Can you work these out from the model? Positions are in its coordinate system, mm. Coordinates: 2 decimals unless noted, no trailing zeros. Order: outer loops, then holes, each group sorted by start corner. A loop starts at its lowest first (then second) coordinate and runs counter-clockwise, first axis right, second up. Notation, with made-up numbers: (58, 74.25) -> (66, 74.25) arc R24 ccw to (66, 101.25) -> close; hole circle Ø8 at (37, 84.25). An arc over 180 degrees is marked (long way). Answer in a Markdown table with one row per item.
Autodesk Inventor part; units mm, degrees
ref_plane "YZ Plane" through (0, 0, 0) normal (1, 0, 0) x (0, 1, 0)
ref_plane "XZ Plane" through (0, 0, 0) normal (0, 1, 0) x (-1, 0, 0)
ref_plane "XY Plane" through (0, 0, 0) normal (0, 0, 1) x (1, 0, 0)
sketch "Szkic1" plane through (0, 0, 0) normal (0, 0, 1) x (1, 0, 0)
  arc A0 (-870, 0) -> (870, 0) centre (0, 0) ccw
  line L0 (-870, 0) -> (870, 0)
  dimension "d0" = 1740
extrude "Płyta1" add sketch "Szkic1" along normal blind 3
sketch "Szkic2" plane through (0, 0, 3) normal (0, 0, 1) x (1, 0, 0)
  circle A0 centre (-780, -80) radius 25
  arc A1 (-870, 0) -> (870, 0) centre (0, 0) ccw
  dimension "d2" = 50
  dimension "d3" = 80
  dimension "d4" = 780
extrude "Wyciągnięcie proste1" cut sketch "Szkic2" against normal blind 10
chamfer "Faza1" distance 2 angle 45 1 edges at (0, 0, 0)
equation "\"d1\" = Grubość"
equation "\"PromieńGięcia\" = Grubość"
equation "\"SzerokośćGięciaPodcięcia\" = Grubość"
equation "\"GłębokośćGięciaPodcięcia\" = 0.5 * Grubość"
equation "\"RozmiarPodcięciaNarożnika\" = 4 * Grubość"
equation "\"MinimalnaPozostałość\" = 2 * Grubość"
equation "\"PromieńPrzejścia\" = PromieńGięcia"
equation "\"Rozmiar_promienia_Jacobiego\" = PromieńGięcia"
equation "\"Wielk_odstępu\" = Grubość"
properties part number "fllooor22" material "Stal nierdzewna"
(1) Suppose I cut it at C-C (x = 617). Please give me the cut outline in (y, z), and give its area (3 significant figures).
Response values:
| item | result |
|---|---|
| outline | (-613.36, 0) -> (-2, 0) -> (0, 2) -> (0, 3) -> (-613.36, 3) -> close |
| area | 1,840 mm2 |
(2) I need wall thicknesses on line 1 (Y direction, x = -780, z = 2.3); line 2 (Y direction, x = -130.5, z = 2); line 3 (X direction, y = -38.5, z = 2.2). Which ranges of each line are inside material? Lowest first, please. Write a range as [from, to].
Response values:
| item | result |
|---|---|
| line 1 | [-385.36, -105], [-55, 0] |
| line 2 | [-860.16, 0] |
| line 3 | [-869.15, 869.15] |
(3) Suppose I cut it at D-D (z = 0.8). Please give me the cut outline in (x, y), and give its area (3 significant figures).
Response values:
| item | result |
|---|---|
| outline | (-870, -1.2) arc R870 ccw to (870, -1.2) -> close; hole circle Ø50 at (-780, -80) |
| area | 1,180,000 mm2 |
(4) Will these pins go through, and if not, where does the flat tip stop? pin 1 Ø1.5 at (y, z) = (-636.5, 1.5) entering from +X; pin 2 Ø1.5 at (y, z) = (-191, 2.5) entering from +X.
Response values:
| item | result |
|---|---|
| pin 1 | x = 593.9 |
| pin 2 | x = 848.94 |
(5) Suppose I cut it at B-B (x = -780). Please give me the cut outline in (y, z), and give its area (3 significant figures).
Response values:
| item | result |
|---|---|
| outline | (-385.36, 0) -> (-105, 0) -> (-105, 3) -> (-385.36, 3) -> close; (-55, 0) -> (-2, 0) -> (0, 2) -> (0, 3) -> (-55, 3) -> close |
| area | 1,000 mm2 |
(6) We'd pull the mould along Y, two halves only. Please class faces 1 (the flat face through (-12, -333, 0)), 2 (the cylindrical face through (-756.154, -72.491, 1.521)), 3 (the cylindrical face through (19.13, -869.79, 1.48)): +Y half, -Y half, draft (parallel to the pull), parting line (faces both ways), or undercut.
Response values:
| item | result |
|---|---|
| face 1 | draft |
| face 2 | undercut |
| face 3 | -Y half |
(7) Suppose I cut it at A-A (y = -80). Please give me the cut outline in (x, z), and give its area (3 significant figures).
Response values:
| item | result |
|---|---|
| outline | (-866.31, 0) -> (-805, 0) -> (-805, 3) -> (-866.31, 3) -> close; (-755, 0) -> (866.31, 0) -> (866.31, 3) -> (-755, 3) -> close |
| area | 5,050 mm2 |
